Work out the finished part from the listing and answer in its coordinate system (mm). Face numbers are marked on the shaded views. A direction names the side the tool comes from. Give positions to 0.01 mm unless a question says otherwise; leave off trailing zeros. Loops run counter-clockwise (first coordinate to the right, second up) from the corner with the lowest first, then second, coordinate; pieces in that order, holes last. Notation, with made-up numbers: M -37.5,69.25 L -25.5,69.25 A17 ccw -25.5,100.25 Z; hole C 63.25,-23 d9. An arc over 180 degrees is marked long. Write item = value, one per line. Start each with the question number.
1. The mould has two halves that part along Z. Classify the marked faces 4, 5 and 6: released by +Z, released by -Z, zero draft, split by the parting line, or undercut.
2. Flat-ended cylindrical pins translate along their axes: pin 1 Ø5 at (x, z) = (44, 68.5) entering from +Y; pin 2 Ø8 at (x, z) = (-12, 37.5) entering from +Y; pin 3 Ø4 at (y, z) = (-36.5, 55) entering from -X. Find the tip coordinate at first contact, or state that the pin passes through.
3. Section B-B on x = 66 is taken. Determine the outline of the cut face in (y, z).
4. Section D-D on y = 19.5 is taken. Determine the outline of the cut face in (x, z), plus the area to 3 significant figures.
5. Section A-A on z = 46 is taken. Determine the outline of the cut face in (x, y), plus the area to 3 significant figures.
6. Consider L1, parallel to Z at x = 50.8, y = -34.5; L2, parallel to X at y = -12, z = 38; L3, parallel to Y at x = 84.5, z = 35. Determine where each line is inside the solid, lowest interval first. Write a range as [from, to].
7. For the marked faces 1, 2 and 3, determine the directions among +Z, -Z, +X, -X, +Y, -Y from which every point of the face is accessible in a straight line to the end or side of a thin tool.
8. Section C-C on z = 69 is taken. Determine the outline of the cut face in (x, y).
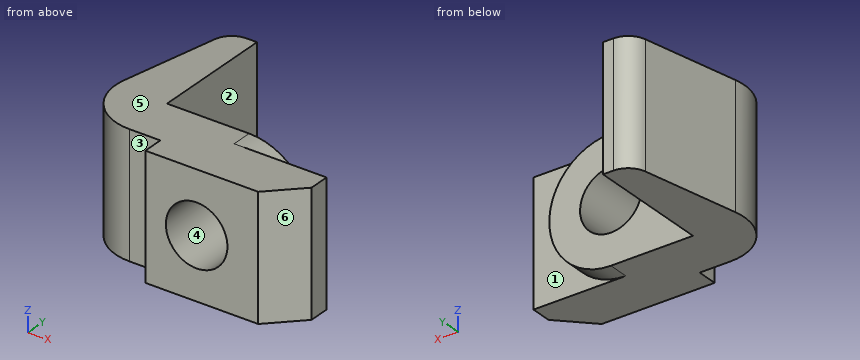
Autodesk Inventor part; units mm, degrees
ref_plane "YZ Plane" through (0, 0, 0) normal (1, 0, 0) x (0, 1, 0)
ref_plane "XZ Plane" through (0, 0, 0) normal (0, 1, 0) x (-1, 0, 0)
ref_plane "XY Plane" through (0, 0, 0) normal (0, 0, 1) x (1, 0, 0)
sketch "Sketch1" plane through (0, 0, 0) normal (0, 0, 1) x (1, 0, 0)
  line L0 (0, 76.2) -> (0, 0)
  line L1 (0, 0) -> (50.8, 0)
  line L2 (50.8, 0) -> (50.8, -12.7)
  line L3 (50.8, -12.7) -> (107.95, -12.7)
  line L4 (107.95, -12.7) -> (107.95, -25.4)
  line L5 (107.95, -25.4) -> (88.9, -44.45)
  line L6 (88.9, -44.45) -> (19.05, -44.45)
  line L7 (0, 76.2) -> (-6.35, 76.2)
  circle A0 centre (-6.35, 63.5) radius 12.7
  circle A1 centre (0, 0) radius 31.75
  line L8 (19.05, -44.45) -> (19.05, -31.75)
  line L9 (-31.0951, 6.4155) -> (-18.788, 66.0662)
  line L10 (19.05, -31.75) -> (0, -31.75)
  point P0 (0, 74.4985)
  dimension "d0" = 6.35
  dimension "d1" = 69.85
  dimension "d2" = 12.7
  dimension "d3" = 76.2
  dimension "d4" = 63.5
  dimension "d5" = 19.05
  dimension "d7" = 31.75
  dimension "d8" = 107.95
  dimension "d9" = 25.4
  dimension "d10" = 12.7
  dimension "d11" = 50.8
  dimension "d12" = 44.45
extrude "Extrusion1" add sketch "Sketch1" along normal blind 76.2 contours L0 A0 L7 | L0 A0 | L0 A1 L9 A0 | L0 L1 A1 | L1 L2 L3 L4 L5 L6 L8 L10 A1 picked at (-6.7952, 59.4597) picked at (-19.9789, 6.5634)
sketch "Sketch2" plane through (50.8, -12.7, 0) normal (0, 1, 0) x (1, 0, 0)
  line L0 (0, 0) -> (0, -76.2) construction
  circle A0 centre (0, -38.1) radius 38.1
  point P0 (-50.8, 0)
extrude "Extrusion2" add sketch "Sketch2" along normal up to surface (12.7 mm away)
sketch "Sketch3" plane through (0, 0, 76.2) normal (0, 1, 0) x (1, 0, 0)
  arc A0 (50.8, 0) -> (50.8, 76.2) centre (50.8, 38.1) ccw construction
  point P0 (0, 76.2)
hole "Hole1" at (50.8, 0, 38.1) direction (0, -1, 0) diameter 38.1 end through all
properties part number "ch4-3"
Verdict:
q1.face_4 = undercut
q1.face_5 = released by +Z
q1.face_6 = zero draft
q2.pin_1 = 0
q2.pin_2 = 76.09
q2.pin_3 = 19.05
q3.outline = M -44.45,0 L -12.7,0 L -12.7,3.16 L 0,3.16 L 0,26.62 L -44.45,26.62 Z; M -44.45,49.58 L 0,49.58 L 0,73.04 L -12.7,73.04 L -12.7,76.2 L -44.45,76.2 Z
q4.outline = M -28.4,0 L 0,0 L 0,76.2 L -28.4,76.2 Z
q4.area = 2,160 mm2
q5.outline = M -31.1,6.42 A31.75 ccw 0,-31.75 L 19.05,-31.75 L 19.05,-44.45 L 33.47,-44.45 L 33.47,0 L 0,0 L 0,76.2 L -6.35,76.2 A12.7 ccw -18.79,66.07 Z; M 68.13,-44.45 L 88.9,-44.45 L 107.95,-25.4 L 107.95,-12.7 L 88.07,-12.7 L 88.07,0 L 68.13,0 Z
q5.area = 5,220 mm2
q6.L1 = [0, 19.05], [57.15, 76.2]
q6.L2 = [-29.39, 31.75], [69.85, 88.9]
q6.L3 = [-44.45, 0]
q7.face_1 = +X, +Y
q7.face_2 = +Z, -Z, +X, +Y
q7.face_3 = +Z, -Z, -X, -Y
q8.outline = M -31.1,6.42 A31.75 ccw 0,-31.75 L 19.05,-31.75 L 19.05,-44.45 L 88.9,-44.45 L 107.95,-25.4 L 107.95,-12.7 L 73.09,-12.7 L 73.09,0 L 0,0 L 0,76.2 L -6.35,76.2 A12.7 ccw -18.79,66.07 Z
